Design review of the part built by this model. Coordinates are the model's own, in mm. A direction names the side the tool comes from. Coordinates: 2 decimals unless noted, no trailing zeros. Loops run counter-clockwise (first coordinate to the right, second up) from the corner with the lowest first, then second, coordinate; pieces in that order, holes last. Notation, with made-up numbers: (26, 14.25) - (55, 14.25) arc R11 cw to (55, 35.25) - close; hole circle Ø2 at (68.25, 63). An arc over 180 degrees is marked (long way). Use one line per item in the form item = value. Start each with the question number.
(1) Tool access review of faces 4 (the face through (-22.21, 102.91, 53.53)), 5 (the face through (22.21, 102.91, 53.53)), 6 (the face through (30, -2, 50)): name each direction out of +Z, -Z, +X, -X, +Y, -Y from which nothing blocks a thin tool from reaching the whole face with its end or side.
(2) Add section C-C (x = -23). State the section outline as (y, z) points.
(3) Add section A-A (z = 0). State the section outline as (x, y) points.
(4) The part is to be moulded in two halves that separate along Y. For faces 1 (the face through (13.993, 113.668, -25.241)), 2 (the face through (-30, -2, 50)), 3 (the face through (-15, 0, 0)), say which applies: pulls with the +Y half, pulls with the -Y half, needs draft (parallel to the pull), parting line crosses it, or undercut.
(5) For L1, parallel to Z at x = -20.5, y = 8; L2, parallel to X at y = -25, z = 4; L3, parallel to X at y = -93, z = -81.5, list the stretches that pass through material, from the lowest coordinate up.
(6) Clearance check with flat-ended pins moving along their axes: pin 1 Ø6 at (x, y) = (21, 95.5) entering from -Z; pin 2 Ø8 at (x, z) = (-19.5, -16.5) entering from -Y; pin 3 Ø4 at (x, z) = (7.5, 54.5) entering from -Y. State where each tip first meets the part, or that it passes through.
```python
from build123d import *


with BuildPart() as part:
    # Sketch1 → Revolve1 (revolve)
    with BuildSketch(Plane.XY, mode=Mode.PRIVATE) as revolve1_sk:
        Polygon((0, 0), (0, 125), (-10, 125), (-14.196768923, 116), (-30, 116), (-30, 45), (-15, 30), (-15, 0), align=None)
    revolve(revolve1_sk.sketch.rotate(Axis((0, 0, 0), (1, 0, 0)), 90), axis=Axis((0, 0, 0), (1, 0, 0)))

    # Mirror1: part across plane


with BuildPart() as part_1:
    add(part.part)
    add(part.part.mirror(Plane.ZY))


solid = part_1.part
```
Computed values:
q1.face_4 = -X
q1.face_5 = +X
q1.face_6 = +Z, -Z, +X, +Y, -Y
q2.outline = circle Ø232 at (0, 0); hole circle Ø76 at (0, 0)
q3.outline = (-30, -116) - (-14.2, -116) - (-10, -125) - (10, -125) - (14.2, -116) - (30, -116) - (30, -45) - (15, -30) - (15, 30) - (30, 45) - (30, 116) - (14.2, 116) - (10, 125) - (-10, 125) - (-14.2, 116) - (-30, 116) - (-30, 45) - (-15, 30) - (-15, -30) - (-30, -45) - close
q4.face_1 = parting line crosses it
q4.face_2 = needs draft
q4.face_3 = undercut
q5.L1 = -115.72 to -34.59, 34.59 to 115.72
q5.L2 = -15 to 15
q5.L3 = -10.63 to 10.63
q6.pin_1 = -70
q6.pin_2 = -115.32
q6.pin_3 = -113.44
